Geometry: see drawing. Coordinates: mm, zero at the bounding-box minimum. A direction names the side the tool comes from. Coordinates: 2 decimals unless noted, no trailing zeros. Order: outer loops, then holes, each group sorted by start corner. A loop starts at its lowest first (then second) coordinate and runs counter-clockwise, first axis right, second up.
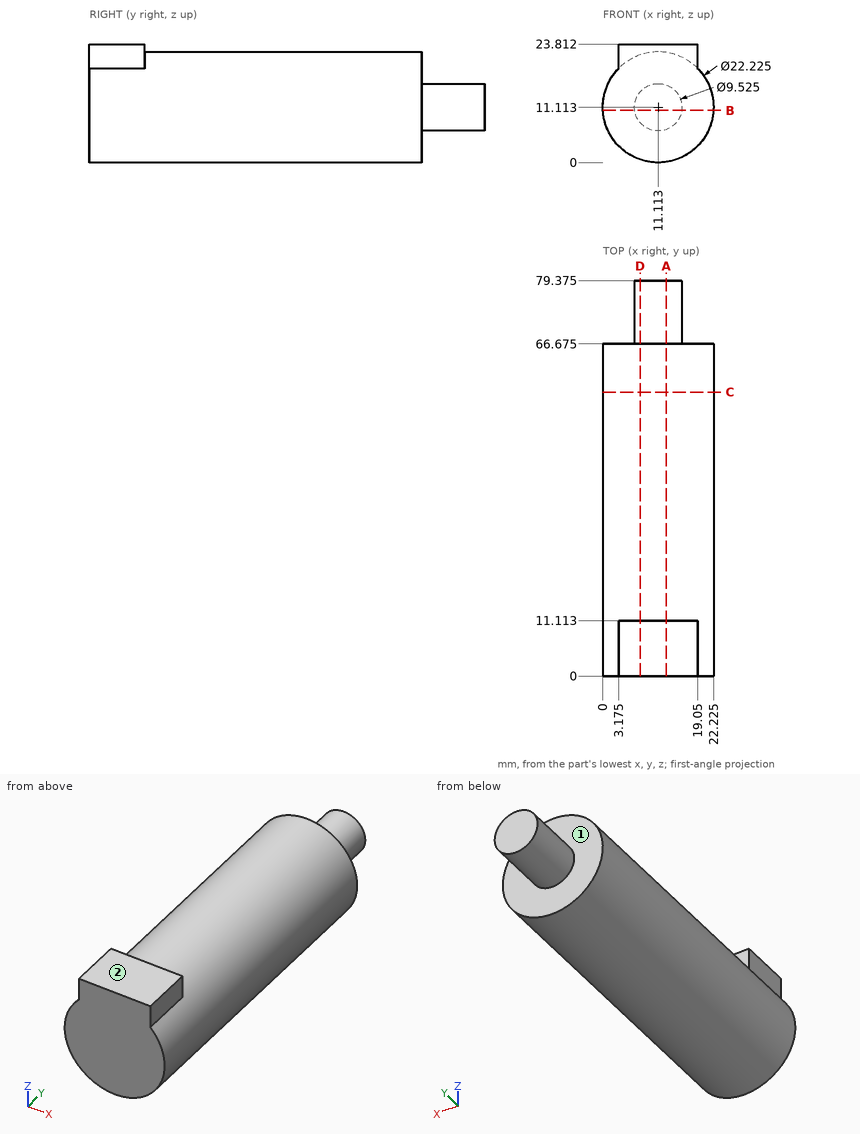
Item 1: Cut plane A-A on x = 12.75. Return loops of the section in (y, z) (1 decimal), then the cut area to 3 significant figures.
Response values:
outline: (0, 0.1) - (66.7, 0.1) - (66.7, 6.6) - (79.4, 6.6) - (79.4, 15.6) - (66.7, 15.6) - (66.7, 22.1) - (11.1, 22.1) - (11.1, 23.8) - (0, 23.8) - close
area: 1,600 mm2
Item 2: Cut plane C-C on y = 57. Return loops of the section in (x, z) (1 decimal).
Response values:
outline: circle Ø22.2 at (11.1, 11.1)
Item 3: Pin query (flat end, axial travel): pin 1 Ø1.5 at (x, y) = (13, 27) entering from -Z; pin 2 Ø2 at (y, z) = (25.5, 12.5) entering from -X; pin 3 Ø5 at (x, z) = (19, 15.5) entering from +Y (1 decimal). Return the tip coordinate at first contact, or that it passes through.
Response values:
pin 1: stops at z = 0.06
pin 2: stops at x = 0.01
pin 3: stops at y = 66.7
Item 4: Ray query, probe 1 along Y at (x, z) = (6.25, 20) (1 decimal); probe 2 along X at (y, z) = (15, 10.5); probe 3 along Z at (x, y) = (11.25, 27.5) (1 decimal). Return the intervals inside material, ascending.
Response values:
probe 1: y = 0 to 66.7
probe 2: x = 0.02 to 22.21
probe 3: z = 0 to 22.2
Item 5: Cut plane B-B on z = 10.5. Return loops of the section in (x, y) (1 decimal), then the cut area to 3 significant figures.
Response values:
outline: (0, 0) - (22.2, 0) - (22.2, 66.7) - (15.8, 66.7) - (15.8, 79.4) - (6.4, 79.4) - (6.4, 66.7) - (0, 66.7) - close
area: 1,600 mm2
Item 6: Cut plane D-D on x = 7.5. Return loops of the section in (y, z) (1 decimal).
Response values:
outline: (0, 0.6) - (66.7, 0.6) - (66.7, 8) - (79.4, 8) - (79.4, 14.2) - (66.7, 14.2) - (66.7, 21.6) - (11.1, 21.6) - (11.1, 23.8) - (0, 23.8) - close
Item 7: Access query for the marked faces 1 and 2. Directions: +Z, -Z, +X, -X, +Y, -Y. A direction counts if a zero-diameter tool reaches every point of the face in a straight line with its end or side. Return the directions, or none.
Response values:
face 1: +Y
face 2: +Z, +X, -X, +Y, -Y
